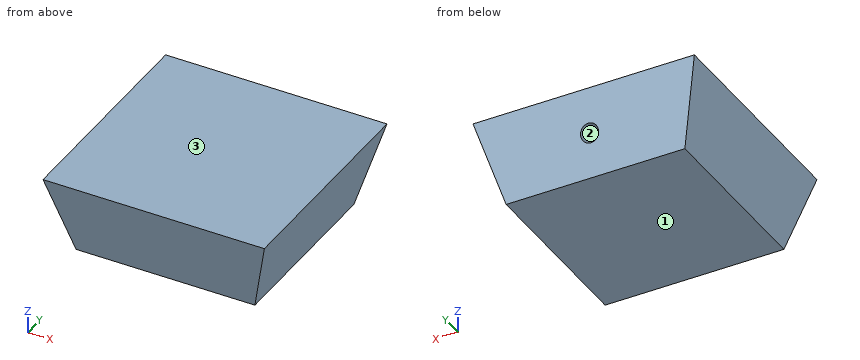
```python
from build123d import *

# Parameters (mm, degrees)
ESQUISSE1_W             = 33.274
ESQUISSE1_H             = 33.274
BOSS_EXTRU_1_DEPTH      = 14.81582
BOSS_EXTRU_1_DRAFT      = -15
ESQUISSE2_R             = 1.666875
ENL_V_MAT_EXTRU_1_DEPTH = 12.7


with BuildPart() as part:
    # Esquisse1 → Boss.-Extru.1 (with draft: the straight prism first)
    with BuildSketch(Plane.XY):
        Rectangle(ESQUISSE1_W, ESQUISSE1_H)
    extrude(amount=BOSS_EXTRU_1_DEPTH)
    # Boss.-Extru.1: the draft: its side faces are tilted about the plane it starts from
    boss_extru_1_sides = [part.faces().sort_by_distance(p)[0] for p in [
        (0, -16.637, 7.40791),
        (16.637, 0, 7.40791),
        (0, 16.637, 7.40791),
        (-16.637, 0, 7.40791),
    ]]
    draft(boss_extru_1_sides, Plane.XY, BOSS_EXTRU_1_DRAFT)

    # Esquisse2 → Enl_v. mat.-Extru.1 (cut)
    with BuildSketch(Plane(origin=(0, 20.32, 0), x_dir=(1, 0, 0), z_dir=(0, 1, 0))):
        with Locations(Location((0, -7.40791, 0), (0, 0, 270))):
            Circle(ESQUISSE2_R)
    extrude(amount=-ENL_V_MAT_EXTRU_1_DEPTH, mode=Mode.SUBTRACT)


solid = part.part
```
Model file for the job. Use its own axes, mm. Face numbers are marked on the shaded views. Coordinates: 2 decimals unless noted, no trailing zeros. Write each loop counter-clockwise with the first axis right and the second up, starting at its lowest first coordinate (ties: lowest second). Pieces come first, ordered by that corner, then holes. Notation, with made-up numbers: (68.25, -38.5) - (117.25, -38.5) arc R20 cw to (117.25, -31.5) - close; hole circle Ø10 at (35, 83.5). An arc over 180 degrees is marked (long way). One line per item, written item: value. Start each with the question number.
1. Mould opens along Z. For the marked faces 1, 2 and 3 say: released by +Z, released by -Z, zero draft, split by the parting line, or undercut.
2. Slice it at A-A (y = 10). Write the cut outline in (x, z), plus the area to 3 significant figures.
3. Slice it at B-B (x = 0). Write the cut outline in (y, z).
4. Probe line 1 (Z direction, x = 0, y = 16); line 2 (Y direction, x = -12.5, z = 11); line 3 (X direction, y = 14.5, z = 7). List the from-to ranges inside material, lowest first. Write a range as from..to.
5. Slice it at C-C (z = 12). Write the cut outline in (x, y).
6. Flat gauge pins, fed straight in: pin 1 (4 mm diameter, centred on x = 9, z = 7, fed in from -Y); pin 2 (2 mm diameter, centred on x = 0, z = 7.41, fed in from +Y); pin 3 (6 mm diameter, centred on y = -7.5, z = 9, fed in from +X); pin 4 (10 mm diameter, centred on x = -16.5, y = 13.5, fed in from -Z). Where does each tip first touch, or does it go through?
7. Slice it at D-D (y = -15.5). Write the cut outline in (x, z).
Answers below:
1. face 1: released by -Z
1. face 2: undercut
1. face 3: released by +Z
2. outline: (-20.61, 14.82) - (-16.64, 0) - (16.64, 0) - (20.61, 14.82) - close; hole circle Ø3.33 at (0, 7.41)
2. area: 543 mm^2
3. outline: (-20.61, 14.82) - (-16.64, 0) - (16.64, 0) - (18.18, 5.74) - (7.62, 5.74) - (7.62, 9.07) - (19.07, 9.07) - (20.61, 14.82) - close
4. line 1: z = 0..5.74, 9.07..14.82
4. line 2: y = -19.58..19.58
4. line 3: x = -18.51..-1.62, 1.62..18.51
5. outline: (-19.85, -19.85) - (19.85, -19.85) - (19.85, 19.85) - (-19.85, 19.85) - close
6. pin 1: stops at y = -19.05
6. pin 2: stops at y = 7.62
6. pin 3: stops at x = 19.85
6. pin 4: stops at z = 0
7. outline: (-20.61, 14.82) - (-16.64, 0) - (16.64, 0) - (20.61, 14.82) - close
